```python
from build123d import *

# Parameters (mm, degrees)
SKETCH1_W            = 20
SKETCH1_H            = 20
BOSS_EXTRUDE1_DEPTH  = 4
CUT_EXTRUDE1_DEPTH   = 2
SKETCH4_W            = 20
SKETCH4_H            = 4
BOSS_EXTRUDE2_DEPTH  = 4
SKETCH5_W            = 4
SKETCH5_H            = 20
BOSS_EXTRUDE3_DEPTH  = 20
CUT_EXTRUDE2_DEPTH   = 2
CUT_EXTRUDE3_DEPTH   = 2
EXTRUDE_THIN2_DEPTH  = 3.5
FILLET1_R            = 1
FILLET1_OF_MIRROR3_R = 1


with BuildPart() as part:
    # Sketch1 → Boss-Extrude1 (new body)
    with BuildSketch(Plane(origin=(0, 0, 0), x_dir=(1, 0, 0), z_dir=(0, 1, 0))):
        Rectangle(SKETCH1_W, SKETCH1_H)
        with BuildLine():
            Line((-4, 2), (4, 2))
            ThreePointArc((4, 2), (6, 0), (4, -2))
            Line((4, -2), (-4, -2))
            ThreePointArc((-4, -2), (-6, 0), (-4, 2))
        make_face(mode=Mode.SUBTRACT)
    extrude(amount=BOSS_EXTRUDE1_DEPTH)

    # Sketch3 → Cut-Extrude1 (cut)
    with BuildSketch(Plane(origin=(0, 4, 0), x_dir=(1, 0, 0), z_dir=(0, 1, 0))):
        with BuildLine():
            Line((-5, 3), (5, 3))
            ThreePointArc((5, 3), (8, 0), (5, -3))
            Line((5, -3), (-5, -3))
            ThreePointArc((-5, -3), (-8, 0), (-5, 3))
        make_face()
    extrude(amount=-CUT_EXTRUDE1_DEPTH, mode=Mode.SUBTRACT)

    # Sketch4 → Boss-Extrude2 (add)
    with BuildSketch(Plane(origin=(10, 0, 0), x_dir=(0, 0, -1), z_dir=(1, 0, 0))):
        with Locations((0, 2)):
            Rectangle(SKETCH4_W, SKETCH4_H)
    extrude(amount=BOSS_EXTRUDE2_DEPTH)

    # Sketch5 → Boss-Extrude3 (add)
    with BuildSketch(Plane(origin=(0, 4, 0), x_dir=(1, 0, 0), z_dir=(0, 1, 0))):
        with Locations((12, 0)):
            Rectangle(SKETCH5_W, SKETCH5_H)
    extrude(amount=BOSS_EXTRUDE3_DEPTH)

    # Sketch6 → Cut-Extrude2 (cut)
    with BuildSketch(Plane.ZY.offset(-10)):
        with BuildLine():
            Line((-3, 9), (-3, 19))
            ThreePointArc((-3, 19), (0, 22), (3, 19))
            Line((3, 19), (3, 9))
            ThreePointArc((3, 9), (0, 6), (-3, 9))
        make_face()
    extrude(amount=-CUT_EXTRUDE2_DEPTH, mode=Mode.SUBTRACT)

    # Sketch7 → Cut-Extrude3 (cut)
    with BuildSketch(Plane.ZY.offset(-12)):
        with BuildLine():
            Line((-2, 10), (-2, 18))
            ThreePointArc((-2, 18), (0, 20), (2, 18))
            Line((2, 18), (2, 10))
            ThreePointArc((2, 10), (0, 8), (-2, 10))
        make_face()
    extrude(amount=-CUT_EXTRUDE3_DEPTH, mode=Mode.SUBTRACT)

    # Sketch17 → Extrude-Thin2 (add)
    with BuildSketch(Plane.XY.offset(-6.5)):
        Polygon((10, 4), (0, 4), (10, 14), align=None)
        Polygon((9, 5), (2.414213562, 5), (9, 11.585786438), align=None, mode=Mode.SUBTRACT)
    extrude_thin2 = extrude(amount=-EXTRUDE_THIN2_DEPTH)

    # Fillet1
    fillet1_edges = [part.edges().sort_by_distance(p)[0] for p in [
        (9, 5, -8.25),
        (2.414213562, 5, -8.25),
        (9, 11.585786438, -8.25),
    ]]
    fillet(fillet1_edges, radius=FILLET1_R)

    # Mirror3: Extrude-Thin2 across plane
    add(extrude_thin2.mirror(Plane.XY))

    # Fillet1 of Mirror3
    fillet1_of_mirror3_edges = [part.edges().sort_by_distance(p)[0] for p in [
        (9, 5, 8.25),
        (2.414213562, 5, 8.25),
        (9, 11.585786438, 8.25),
    ]]
    fillet(fillet1_of_mirror3_edges, radius=FILLET1_OF_MIRROR3_R)


solid = part.part
```
Model file for the job. Use its own axes, mm. A direction names the side the tool comes from. Coordinates: 2 decimals unless noted, no trailing zeros. Order: outer loops, then holes, each group sorted by start corner. A loop starts at its lowest first (then second) coordinate and runs counter-clockwise, first axis right, second up. Notation, with made-up numbers: (32.25, -34.75) -> (42.25, -34.75) arc R28 ccw to (42.25, -7.75) -> close; hole circle Ø9 at (42.5, 85). An arc over 180 degrees is marked (long way). Return JSON: item names as keys, results as strings.
Item 1: Mould opens along Z. For faces 1 (the face through (5.685, 8.271, 8.226)), 2 (the face through (13, 14, -2)) say: pulls with the +Z half, pulls with the -Z half, needs draft (parallel to the pull), parting line crosses it, or undercut.
Model answer:
{"face 1": "needs draft", "face 2": "undercut"}
Item 2: Slice it at A-A (x = 6.75). Write the cut outline in (y, z), then the cut area to 3 significant figures.
Model answer:
{"outline": "(0, -10) -> (5, -10) -> (5, -6.5) -> (4, -6.5) -> (4, -2.44) -> (2, -2.44) -> (2, 2.44) -> (4, 2.44) -> (4, 6.5) -> (5, 6.5) -> (5, 10) -> (0, 10) -> close; (9.34, -10) -> (10.75, -10) -> (10.75, -6.5) -> (9.34, -6.5) -> close; (9.34, 6.5) -> (10.75, 6.5) -> (10.75, 10) -> (9.34, 10) -> close", "area": "87.2 mm²"}
Item 3: 3-axis set-ups, long thin cutter, end or side, ignore diameter. For faces 3 (the face through (-6, 1, 0)), 4 (the face through (6, 5, -8)), 5 (the face through (5, 8, 6.5)): which of +Z, -Z, +X, -X, +Y, -Y reach the whole face in a straight line?
Model answer:
{"face 3": "+Y, -Y", "face 4": "+Z, -Z", "face 5": "-X, +Y"}
Item 4: Slice it at B-B (z = 0). Write the cut outline in (x, y), then the cut area to 3 significant figures.
Model answer:
{"outline": "(-10, 0) -> (-6, 0) -> (-6, 2) -> (-8, 2) -> (-8, 4) -> (-10, 4) -> close; (6, 0) -> (14, 0) -> (14, 8) -> (12, 8) -> (12, 6) -> (10, 6) -> (10, 4) -> (8, 4) -> (8, 2) -> (6, 2) -> close; (10, 22) -> (12, 22) -> (12, 20) -> (14, 20) -> (14, 24) -> (10, 24) -> close", "area": "64.0 mm²"}
Item 5: Slice it at C-C (y = 5.5). Write the cut outline in (x, z), then the cut area to 3 significant figures.
Model answer:
{"outline": "(1.5, -10) -> (3.96, -10) -> (3.96, -6.5) -> (1.5, -6.5) -> close; (1.5, 6.5) -> (3.96, 6.5) -> (3.96, 10) -> (1.5, 10) -> close; (8.87, -10) -> (14, -10) -> (14, 10) -> (8.87, 10) -> (8.87, 6.5) -> (10, 6.5) -> (10, -6.5) -> (8.87, -6.5) -> close", "area": "105 mm²"}
Item 6: Wall check: line 1 along Z through (x, y) = (9.75, 13); line 2 along Y through (x, z) = (-8.25, -1); line 3 along X through (y, z) = (16.75, 7). Give the ranges that are in metal, low to high. Write a range as from..to.
Model answer:
{"line 1": "z = -10..-6.5, 6.5..10", "line 2": "y = 0..4", "line 3": "x = 10..14"}
Item 7: Pin check, flat tips, straight feed: P1, Ø6, axis at y = 11, z = -4, coming from the -X side; P2, Ø12, axis at y = 18.5, z = -1, coming from the -X side; P3, Ø1.6, axis at y = 8, z = -9, coming from the -X side. Stop position of each tip, or through.
Model answer:
{"P1": "stops at x = 5.34", "P2": "stops at x = 10", "P3": "stops at x = 3.2"}
